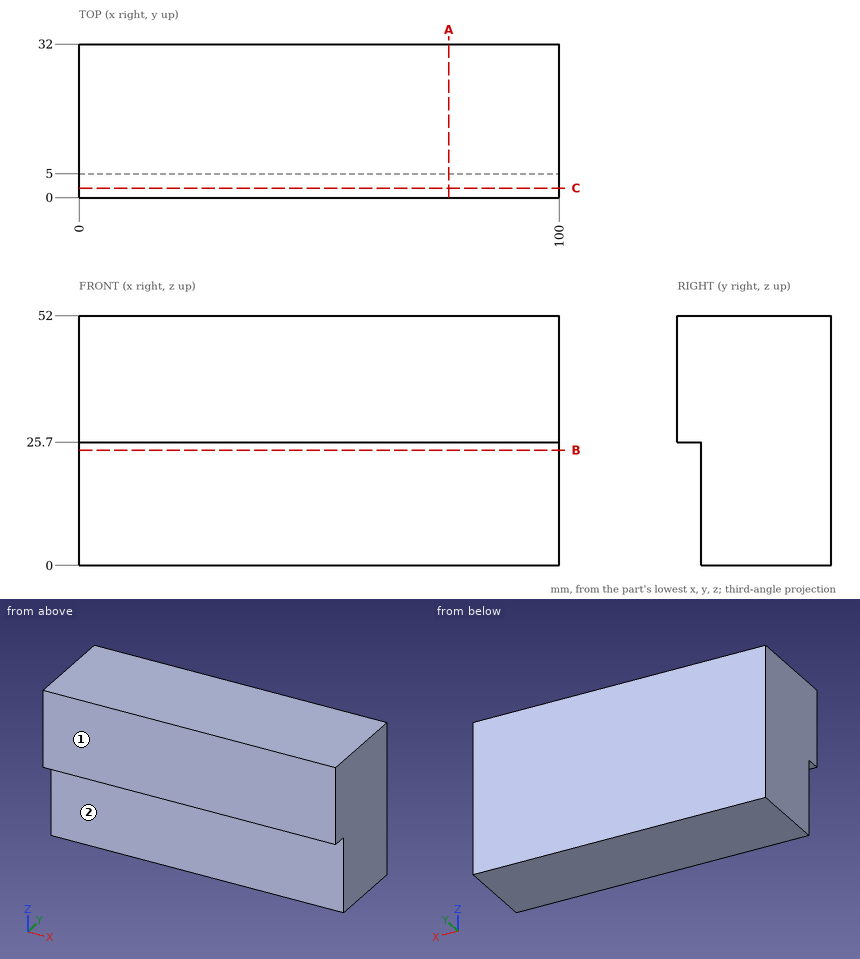
Here's the drawing with two shaded views (mm, measured from the low corner). I have some questions. A direction names the side the tool comes from. Give positions to 0.01 mm unless a question says otherwise; leave off trailing zeros. Loops run counter-clockwise (first coordinate to the right, second up) from the corner with the lowest first, then second, coordinate; pieces in that order, holes last. Notation, with made-up numbers: (63.25, 64.5) -> (79.25, 64.5) arc R13 ccw to (79.25, 84.5) -> close; hole circle Ø3 at (-20.5, 48). An arc over 180 degrees is marked (long way). Answer as a JSON object with one key per item and string values. Group by question number.
Item 1: I need wall thicknesses on L1, parallel to Y at x = 54, z = 10.5. Which ranges of the line are inside material? Lowest first, please.
Item 2: Imagine slicing it at A-A on x = 77. Write out the boundary of the cut face in (y, z).
Item 3: Imagine slicing it at B-B on z = 24. Write out the boundary of the cut face in (x, y), then the cut area to 3 significant figures.
Item 4: On a 3-axis mill with a long thin cutter (end or side, diameter ignored), from which of +Z, -Z, +X, -X, +Y, -Y can I reach the whole of each face in a straight line? I mean the marked faces 1 and 2. Say none if no direction works.
Item 5: Imagine slicing it at C-C on y = 2. Write out the boundary of the cut face in (x, z).
Item 6: Will these pins go through, and if not, where does the flat tip stop? pin 1 (5.5 mm diameter, centred on x = 41, y = 1.5, fed in from -Z); pin 2 (20.5 mm diameter, centred on x = 52, z = 6.5, fed in from -Y).
Answer list:
{
 "1": {"L1": "y = 5 to 32"},
 "2": {"outline": "(0, 25.7) -> (5, 25.7) -> (5, 0) -> (32, 0) -> (32, 52) -> (0, 52) -> close"},
 "3": {"outline": "(0, 5) -> (100, 5) -> (100, 32) -> (0, 32) -> close", "area": "2,700 mm2"},
 "4": {"face 1": "+Z, -Z, +X, -X, -Y", "face 2": "-Z, +X, -X, -Y"},
 "5": {"outline": "(0, 25.7) -> (100, 25.7) -> (100, 52) -> (0, 52) -> close"},
 "6": {"pin 1": "stops at z = 25.7", "pin 2": "stops at y = 5"}
}
